Source: CAD feature listing. Evaluate the final solid. Frame: model axes, mm. Face numbers are marked on the shaded views. A direction names the side the tool comes from. Give positions to 0.01 mm unless a question says otherwise; leave off trailing zeros. Loops run counter-clockwise (first coordinate to the right, second up) from the corner with the lowest first, then second, coordinate; pieces in that order, holes last. Notation, with made-up numbers: M 38,6.5 L 76,6.5 A35 cw 76,38.5 Z; hole C 6,17.25 d9. An arc over 180 degrees is marked long. Answer in a Markdown table with one row per item.
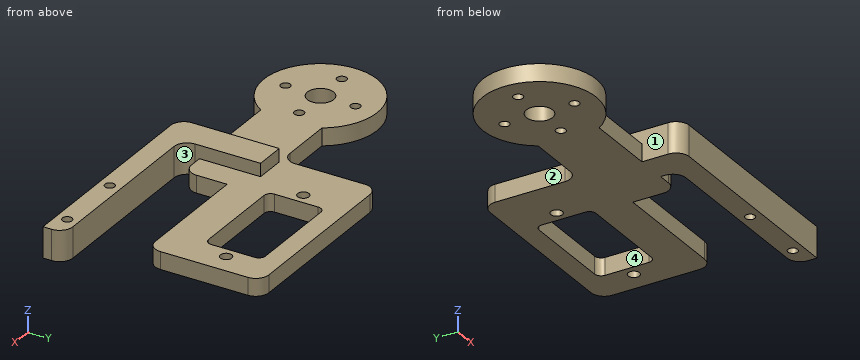
```python
from build123d import *

# Parameters (mm, degrees)
ELBOW_HORN_FLANGE_PROFILE_R          = 13
ELBOW_HORN_FLANGE_DEPTH              = 4
FOREARM_WEB_PROFILE_W                = 40
FOREARM_WEB_PROFILE_H                = 14
FOREARM_WEB_DEPTH                    = 4
GRIPPER_SERVO_MOUNT_PROFILE_W        = 44
GRIPPER_SERVO_MOUNT_PROFILE_H        = 26
GRIPPER_SERVO_MOUNT_DEPTH            = 4
GRIP_SG90_BODY_CLEARANCE_START       = -5
GRIP_SG90_BODY_CLEARANCE_PROFILE_W   = 23.8
GRIP_SG90_BODY_CLEARANCE_PROFILE_H   = 13
GRIP_SG90_BODY_CLEARANCE_DEPTH       = 81.874897035
GRIP_SERVO_TAB_FASTENERS_START       = -50
GRIP_SERVO_TAB_FASTENERS_PROFILE_R   = 1.3
GRIP_SERVO_TAB_FASTENERS_DEPTH       = 126.874897035
FIXED_FINGER_SPINE_PROFILE_W         = 48
FIXED_FINGER_SPINE_PROFILE_H         = 5
FIXED_FINGER_SPINE_DEPTH             = 7
FIXED_FINGER_ROOT_PROFILE_W          = 7
FIXED_FINGER_ROOT_PROFILE_H          = 23
FIXED_FINGER_ROOT_DEPTH              = 7
ELBOW_CENTER_SCREW_ACCESS_START      = -50
ELBOW_CENTER_SCREW_ACCESS_PROFILE_R  = 3
ELBOW_CENTER_SCREW_ACCESS_DEPTH      = 134.510478384
ELBOW_HORN_FASTENERS_START           = -50
ELBOW_HORN_FASTENERS_PROFILE_R       = 1.1
ELBOW_HORN_FASTENERS_DEPTH           = 134.510478384
FIXED_PAD_KEEPER_FASTENERS_START     = -50
FIXED_PAD_KEEPER_FASTENERS_PROFILE_R = 1.1
FIXED_PAD_KEEPER_FASTENERS_DEPTH     = 134.510478384
FILLET1_R                            = 3
FILLET2_R                            = 1.5


with BuildPart() as part:
    # Elbow_horn_flange_profile → Elbow_horn_flange (new body)
    with BuildSketch(Plane.XY):
        Circle(ELBOW_HORN_FLANGE_PROFILE_R)
    extrude(amount=ELBOW_HORN_FLANGE_DEPTH)

    # Forearm_web_profile → Forearm_web (add)
    with BuildSketch(Plane.XY):
        with Locations((20, 0)):
            Rectangle(FOREARM_WEB_PROFILE_W, FOREARM_WEB_PROFILE_H)
    extrude(amount=FOREARM_WEB_DEPTH)

    # Gripper_servo_mount_profile → Gripper_servo_mount (add)
    with BuildSketch(Plane.XY):
        with Locations((48, 16)):
            Rectangle(GRIPPER_SERVO_MOUNT_PROFILE_W, GRIPPER_SERVO_MOUNT_PROFILE_H)
    extrude(amount=GRIPPER_SERVO_MOUNT_DEPTH)

    # Grip_SG90_body_clearance_profile → Grip_SG90_body_clearance (cut, through all)
    with BuildSketch(Plane.XY.offset(GRIP_SG90_BODY_CLEARANCE_START)):
        with Locations((50.5, 18)):
            Rectangle(GRIP_SG90_BODY_CLEARANCE_PROFILE_W, GRIP_SG90_BODY_CLEARANCE_PROFILE_H)
    extrude(amount=GRIP_SG90_BODY_CLEARANCE_DEPTH, mode=Mode.SUBTRACT)

    # Grip_servo_tab_fasteners_profile → Grip_servo_tab_fasteners (cut, through all)
    with BuildSketch(Plane.XY.offset(GRIP_SERVO_TAB_FASTENERS_START)):
        with Locations((36, 18)):
            Circle(GRIP_SERVO_TAB_FASTENERS_PROFILE_R)
        with Locations((65, 18)):
            Circle(GRIP_SERVO_TAB_FASTENERS_PROFILE_R)
    extrude(amount=GRIP_SERVO_TAB_FASTENERS_DEPTH, mode=Mode.SUBTRACT)



with BuildPart() as body_2:
    # Fixed_finger_spine_profile → Fixed_finger_spine (new body)
    with BuildSketch(Plane.XY):
        with Locations((54, -13.5)):
            Rectangle(FIXED_FINGER_SPINE_PROFILE_W, FIXED_FINGER_SPINE_PROFILE_H)
    extrude(amount=FIXED_FINGER_SPINE_DEPTH)


with BuildPart() as part_1:
    add(part.part)

    add(body_2.part)  # Fixed_finger_root merges body 2
    # Fixed_finger_root_profile → Fixed_finger_root (add)
    with BuildSketch(Plane.XY):
        with Locations((30.5, -4.5)):
            Rectangle(FIXED_FINGER_ROOT_PROFILE_W, FIXED_FINGER_ROOT_PROFILE_H)
    extrude(amount=FIXED_FINGER_ROOT_DEPTH)

    # Elbow_center_screw_access_profile → Elbow_center_screw_access (cut, through all)
    with BuildSketch(Plane.XY.offset(ELBOW_CENTER_SCREW_ACCESS_START)):
        with Locations(Location((0, 0, 0), (0, 0, 180))):
            Circle(ELBOW_CENTER_SCREW_ACCESS_PROFILE_R)
    extrude(amount=ELBOW_CENTER_SCREW_ACCESS_DEPTH, mode=Mode.SUBTRACT)

    # Elbow_horn_fasteners_profile → Elbow_horn_fasteners (cut, through all)
    with BuildSketch(Plane.XY.offset(ELBOW_HORN_FASTENERS_START)):
        with Locations(Location((0, -8, 0), (0, 0, 180))):
            Circle(ELBOW_HORN_FASTENERS_PROFILE_R)
        with Locations(Location((0, 8, 0), (0, 0, 180))):
            Circle(ELBOW_HORN_FASTENERS_PROFILE_R)
        with Locations(Location((-8, 0, 0), (0, 0, 180))):
            Circle(ELBOW_HORN_FASTENERS_PROFILE_R)
        with Locations(Location((8, 0, 0), (0, 0, 180))):
            Circle(ELBOW_HORN_FASTENERS_PROFILE_R)
    extrude(amount=ELBOW_HORN_FASTENERS_DEPTH, mode=Mode.SUBTRACT)

    # Fixed_pad_keeper_fasteners_profile → Fixed_pad_keeper_fasteners (cut, through all)
    with BuildSketch(Plane.XY.offset(FIXED_PAD_KEEPER_FASTENERS_START)):
        with Locations(Location((57, -13.5, 0), (0, 0, 180))):
            Circle(FIXED_PAD_KEEPER_FASTENERS_PROFILE_R)
        with Locations(Location((73, -13.5, 0), (0, 0, 180))):
            Circle(FIXED_PAD_KEEPER_FASTENERS_PROFILE_R)
    extrude(amount=FIXED_PAD_KEEPER_FASTENERS_DEPTH, mode=Mode.SUBTRACT)

    # Fillet1
    fillet1_edges = [part_1.edges().sort_by_distance(p)[0] for p in [
        (34, -11, 3.5),
        (78, -11, 3.5),
        (40, -7, 2),
        (26, 7, 2),
        (26, 29, 2),
        (70, 3, 2),
        (70, 29, 2),
        (27, -16, 3.5),
    ]]
    fillet(fillet1_edges, radius=FILLET1_R)

    # Fillet2
    fillet2_edges = [part_1.edges().sort_by_distance(p)[0] for p in [
        (38.6, 24.5, 2),
        (38.6, 11.5, 2),
        (62.4, 11.5, 2),
        (62.4, 24.5, 2),
    ]]
    fillet(fillet2_edges, radius=FILLET2_R)


solid = part_1.part
```
Q1. Ray query, probe 1 along Y at (x, z) = (65, 1.4); probe 2 along X at (y, z) = (18, 1.95); probe 3 along Y at (x, z) = (73, 4.5). Return the intervals inside material, ascending. Write a range as from..to.
Values follow:
| item | result |
|---|---|
| probe 1 | -16..-11, 3..16.7, 19.3..29 |
| probe 2 | 26..34.7, 37.3..38.6, 62.4..63.7, 66.3..70 |
| probe 3 | -16..-14.6, -12.4..-11 |
Q2. Contact query for flat-ended pins moving along their axis: pin 1 Ø1.6 at (x, y) = (65, 18) entering from -Z; pin 2 Ø4 at (x, z) = (27.5, 3) entering from -Y; pin 3 Ø1 at (x, y) = (54, 7.5) entering from +Z; pin 4 Ø1.5 at (x, z) = (19, 4) entering from -Y. Output: stop coordinate, or through.
Values follow:
| item | result |
|---|---|
| pin 1 | through |
| pin 2 | y = -15.96 |
| pin 3 | z = 4 |
| pin 4 | y = -7 |
Q3. Section query C-C (x = 57). Output: boundary loops of the cut face in (y, z).
Values follow:
| item | result |
|---|---|
| outline | M -16,0 L -14.6,0 L -14.6,7 L -16,7 Z; M -12.4,0 L -11,0 L -11,7 L -12.4,7 Z; M 3,0 L 11.5,0 L 11.5,4 L 3,4 Z; M 24.5,0 L 29,0 L 29,4 L 24.5,4 Z |
Q4. Section query A-A (y = 0). Output: boundary loops of the cut face in (x, z), plus the area to 3 significant figures.
Values follow:
| item | result |
|---|---|
| outline | M -13,0 L -9.1,0 L -9.1,4 L -13,4 Z; M -6.9,0 L -3,0 L -3,4 L -6.9,4 Z; M 3,0 L 6.9,0 L 6.9,4 L 3,4 Z; M 9.1,0 L 40,0 L 40,4 L 34,4 L 34,7 L 27,7 L 27,4 L 9.1,4 Z |
| area | 191 mm^2 |
Q5. Reachability of the marked faces 1, 2, 3 and 4 from +Z, -Z, +X, -X, +Y, -Y: full face, straight path, thin tool, end or side. Return the list, or none.
Values follow:
| item | result |
|---|---|
| face 1 | +Z, -Y |
| face 2 | +Z, -Z, +Y |
| face 3 | +Z, -Z, +X |
| face 4 | +Z, -Z |
Q6. Section query D-D (y = 8). Output: boundary loops of the cut face in (x, z).
Values follow:
| item | result |
|---|---|
| outline | M -10.25,0 L -1.1,0 L -1.1,4 L -10.25,4 Z; M 1.1,0 L 10.25,0 L 10.25,4 L 1.1,4 Z; M 25.24,0 L 70,0 L 70,4 L 25.24,4 Z |
Q7. Section query B-B (x = 73). Output: boundary loops of the cut face in (y, z), plus the area to 3 significant figures.
Values follow:
| item | result |
|---|---|
| outline | M -16,0 L -14.6,0 L -14.6,7 L -16,7 Z; M -12.4,0 L -11,0 L -11,7 L -12.4,7 Z |
| area | 19.6 mm^2 |
